from build123d import *

# Parameters (mm, degrees)
CROQUIS1_W              = 210
CROQUIS1_H              = 50
CROQUIS1_R              = 12.5
SALIENTE_EXTRUIR1_DEPTH = 40
REDONDEO1_R             = 5
CORTAR_EXTRUIR1_DEPTH   = 191.91883092


with BuildPart() as part:
    # Croquis1 → Saliente-Extruir1 (new body)
    with BuildSketch(Plane.XY):
        with Locations((80, 0)):
            Rectangle(CROQUIS1_W, CROQUIS1_H)
        Circle(CROQUIS1_R, mode=Mode.SUBTRACT)
    extrude(amount=SALIENTE_EXTRUIR1_DEPTH)

    # Redondeo1
    redondeo1_edges = [part.edges().sort_by_distance(p)[0] for p in [
        (80, 25, 40),
        (-25, 0, 40),
        (80, -25, 40),
        (-25, 0, 0),
        (80, 25, 0),
        (80, -25, 0),
        (-25, -25, 20),
        (-25, 25, 20),
    ]]
    fillet(redondeo1_edges, radius=REDONDEO1_R)

    # Croquis2 → Cortar-Extruir1 (cut, through all)
    with BuildSketch(Plane.XY.offset(40)):
        with BuildLine():
            Line((149.499217678, 10), (35.500782322, 10))
            ThreePointArc((35.500782322, 10), (33.379461979, 9.121320344), (32.500782322, 7))
            Line((32.500782322, 7), (32.500782322, -7))
            ThreePointArc((32.500782322, -7), (33.379461979, -9.121320344), (35.500782322, -10))
            Line((35.500782322, -10), (149.499217678, -10))
            ThreePointArc((149.499217678, -10), (151.620538021, -9.121320344), (152.499217678, -7))
            Line((152.499217678, -7), (152.499217678, 7))
            ThreePointArc((152.499217678, 7), (151.620538021, 9.121320344), (149.499217678, 10))
        make_face()
    extrude(amount=-CORTAR_EXTRUIR1_DEPTH, mode=Mode.SUBTRACT)


solid = part.part
The listing builds one solid part. Answer for the finished solid, in the listing's coordinates (mm). A direction names the side the tool comes from. Coordinates: 2 decimals unless noted, no trailing zeros. Write each loop counter-clockwise with the first axis right and the second up, starting at its lowest first coordinate (ties: lowest second). Pieces come first, ordered by that corner, then holes. Notation, with made-up numbers: (70.5, 74) - (106.5, 74) arc R34 cw to (106.5, 111) - close; hole circle Ø5 at (88, 47). An arc over 180 degrees is marked (long way). Return JSON: item names as keys, results as strings.
1. Which of the six approach directions +Z, -Z, +X, -X, +Y, -Y give full straight-line access (tool end or side, diameter ignored) to faces 1 (the face through (84, 24, 38)), 2 (the face through (32.501, 0, 20))?
Final values:
{"face 1": "+Z, +X, -X, +Y", "face 2": "+Z, -Z"}
2. The part is cut by section D-D on x = 0. Determine the outline of the cut face in (y, z), then the cut area to 3 significant figures.
Final values:
{"outline": "(-25, 5) arc R5 ccw to (-20, 0) - (-12.5, 0) - (-12.5, 40) - (-20, 40) arc R5 ccw to (-25, 35) - close; (12.5, 0) - (20, 0) arc R5 ccw to (25, 5) - (25, 35) arc R5 ccw to (20, 40) - (12.5, 40) - close", "area": "979 mm^2"}
3. The part is cut by section A-A on x = 130.5. Determine the outline of the cut face in (y, z), then the cut area to 3 significant figures.
Final values:
{"outline": "(-25, 5) arc R5 ccw to (-20, 0) - (-10, 0) - (-10, 40) - (-20, 40) arc R5 ccw to (-25, 35) - close; (10, 0) - (20, 0) arc R5 ccw to (25, 5) - (25, 35) arc R5 ccw to (20, 40) - (10, 40) - close", "area": "1,180 mm^2"}
4. For a pull along X with two mould halves and no side action, classify faces 3 (the face through (-24, 23, 20)), 4 (the face through (93, 10, 20)), 5 (the face through (185, 0, 20)), 6 (the face through (84, 24, 2)) as +X half, -X half, draft (parallel to the pull), parting line (faces both ways), or undercut.
Final values:
{"face 3": "-X half", "face 4": "undercut", "face 5": "+X half", "face 6": "draft"}
5. The part is cut by section B-B on y = 0. Determine the outline of the cut face in (x, z), then the cut area to 3 significant figures.
Final values:
{"outline": "(-25, 5) arc R5 ccw to (-20, 0) - (-12.5, 0) - (-12.5, 40) - (-20, 40) arc R5 ccw to (-25, 35) - close; (12.5, 0) - (32.5, 0) - (32.5, 40) - (12.5, 40) - close; (152.5, 0) - (185, 0) - (185, 40) - (152.5, 40) - close", "area": "2,590 mm^2"}
6. Consider line 1 along X through (y, z) = (-0.5, 9); line 2 along Y through (x, z) = (0, 28.5); line 3 along Y through (x, z) = (133.5, 30). Determine where each line is inside the solid, lowest interval first.
Final values:
{"line 1": "-25 to -12.49, 12.49 to 32.5, 152.5 to 185", "line 2": "-25 to -12.5, 12.5 to 25", "line 3": "-25 to -10, 10 to 25"}
7. The part is cut by section C-C on z = 20. Determine the outline of the cut face in (x, y).
Final values:
{"outline": "(-25, -20) arc R5 ccw to (-20, -25) - (185, -25) - (185, 25) - (-20, 25) arc R5 ccw to (-25, 20) - close; hole circle Ø25 at (0, 0); hole (32.5, -7) arc R3 ccw to (35.5, -10) - (149.5, -10) arc R3 ccw to (152.5, -7) - (152.5, 7) arc R3 ccw to (149.5, 10) - (35.5, 10) arc R3 ccw to (32.5, 7) - close"}
